Part model, mm, in its own coordinate system. A direction names the side the tool comes from. Round coordinates to 2 decimals unless told otherwise and drop trailing zeros. Loops run counter-clockwise (first coordinate to the right, second up) from the corner with the lowest first, then second, coordinate; pieces in that order, holes last. Notation, with made-up numbers: (-18, -7) - (8, -7) arc R22 ccw to (8, 8) - close; hole circle Ø2 at (-31, 72). An arc over 180 degrees is marked (long way). Put each result on its own line as item: value.
Autodesk Inventor part; units mm, degrees
ref_plane "YZ Plane" through (0, 0, 0) normal (1, 0, 0) x (0, 1, 0)
ref_plane "XZ Plane" through (0, 0, 0) normal (0, 1, 0) x (-1, 0, 0)
ref_plane "XY Plane" through (0, 0, 0) normal (0, 0, 1) x (1, 0, 0)
sketch "Sketch1" plane through (0, 0, 0) normal (0, 0, 1) x (1, 0, 0)
  line L0 (0, 0) -> (50, 0)
  line L1 (50, 0) -> (50, 150)
  line L2 (50, 150) -> (0, 150)
  line L3 (0, 150) -> (0, 0)
  dimension "d0" = 50
  dimension "d1" = 150
extrude "Plate1" add sketch "Sketch1" along normal blind 1
sketch "Sketch2" plane through (50, 149, 1) normal (0, 1, 0) x (-1, 0, 0)
  line L0 (50, 0) -> (0, 0)
  line L1 (0, 0) -> (0, -79)
  line L2 (0, -79) -> (50, -79)
  line L3 (50, -79) -> (50, 0)
edge flange "Flange1" height 79 angle 90 thickness 1 bend radius 1 thickness toward (0, 1, 0) relief tear relief width 1 relief depth 0.5 edges at (25, 150, 0) wall of the first edge with corners at (0, 149, 1) (50, 149, 1) (50, 149, -78) (0, 149, -78)
bend "Bend1"
corner "Corner1"
sketch "Sketch4" plane through (0, 150, -78) normal (0, 1, 0) x (1, 0, 0)
  line L0 (0, 0) -> (50, 0)
  line L1 (0, 0) -> (-40, 0)
  line L2 (-40, 0) -> (-40, -40)
  line L3 (-40, -40) -> (0, -40)
  line L4 (0, -40) -> (0, 0)
  line L5 (50, -77) -> (50, 0)
  line L6 (50, 0) -> (90, 0)
  line L7 (90, 0) -> (90, -40)
  line L8 (90, -40) -> (50, -40)
  line L9 (50, -40) -> (50, 0)
  point P0 (0, -78)
  dimension "d14" = 40
  dimension "d15" = 40
  dimension "d16" = 40
  dimension "d17" = 40
sheet face with bend "Face2" sketch "Sketch4" thickness 1 toward (0, -1, 0) bend radius 1
bend "Bend2"
fillet "Corner Round7" radius 6 2 edges at (50, 149.5, -38) (0, 149.5, -38)
sketch "Sketch3" plane through (0, 150, -78) normal (0, 1, 0) x (1, 0, 0)
  line L0 (0, 0) -> (50, 0)
  circle A0 centre (25, 0) radius 45.5
  arc A1 (-16.7744, -26.5) -> (66.7744, -26.5) centre (25, 0) ccw
  arc A2 (0, -46) -> (-6, -40) centre (-6, -46) ccw
  circle A3 centre (-6, -46) radius 6
  arc A4 (56, -40) -> (50, -46) centre (56, -46) ccw
  circle A5 centre (56, -46) radius 6
  line L1 (-40, -40) -> (-6, -40)
  line L2 (-6, -40) -> (-40, -40)
  line L3 (-40, 0) -> (-40, -40)
  line L4 (-40, -40) -> (-40, 0)
  line L5 (-40, 0) -> (-20.5, 0)
  line L6 (90, 0) -> (-40, 0)
  line L7 (56, -40) -> (90, -40)
  line L8 (56, -40) -> (90, -40)
  line L9 (90, -40) -> (90, 0)
  line L10 (90, -40) -> (90, 0)
  line L11 (90, 0) -> (70.5, 0)
  line L12 (25, 0) -> (25, -45.5)
  line L13 (25, -45.5) -> (25, -23.5) construction
  line L14 (25, -23.5) -> (63.9615, -23.5) construction
  line L15 (63.9615, -23.5) -> (69.9615, -23.5)
  line L16 (63.9615, -23.5) -> (69.9615, -23.5) construction
  line L17 (71.9615, -25.5) -> (71.9615, -30)
  line L18 (70.4615, -31.5) -> (70.4615, -31.5)
  line L19 (25, -23.5) -> (-13.9615, -23.5) construction
  line L20 (-13.9615, -23.5) -> (-19.9615, -23.5)
  line L21 (-13.9615, -23.5) -> (-7.9615, -23.5) construction
  line L22 (-21.9615, -25.5) -> (-21.9615, -30)
  line L23 (-20.4615, -31.5) -> (-20.4615, -31.5)
  arc A6 (-16.7744, -26.5) -> (66.7744, -26.5) centre (25, 0) ccw
  line L24 (-18.9615, -30) -> (-18.9615, -27.5)
  line L25 (-17.9615, -26.5) -> (-16.7744, -26.5)
  line L26 (68.9615, -30) -> (68.9615, -27.5)
  line L27 (67.9615, -26.5) -> (66.7744, -26.5)
  arc A7 (-19.9615, -23.5) -> (-21.9615, -25.5) centre (-19.9615, -25.5) ccw
  arc A8 (-21.9615, -30) -> (-20.4615, -31.5) centre (-20.4615, -30) ccw
  arc A9 (-20.4615, -31.5) -> (-18.9615, -30) centre (-20.4615, -30) ccw
  arc A10 (-17.9615, -26.5) -> (-18.9615, -27.5) centre (-17.9615, -27.5) ccw
  arc A11 (71.9615, -25.5) -> (69.9615, -23.5) centre (69.9615, -25.5) ccw
  arc A12 (70.4615, -31.5) -> (71.9615, -30) centre (70.4615, -30) ccw
  arc A13 (68.9615, -30) -> (70.4615, -31.5) centre (70.4615, -30) ccw
  arc A14 (68.9615, -27.5) -> (67.9615, -26.5) centre (67.9615, -27.5) ccw
  point P0 (0, -78)
  point P1 (52.6469, -41.0244)
  point P2 (-2.6469, -41.0244)
  point P3 (71.9615, -23.5)
  point P4 (71.9615, -31.5)
  point P5 (68.9615, -31.5)
  point P6 (-21.9615, -23.5)
  point P7 (-21.9615, -31.5)
  point P8 (-18.9615, -31.5)
  point P9 (-18.9615, -26.5)
  point P10 (68.9615, -26.5)
  point P11 (-2.6469, -41.0244)
  point P12 (52.6469, -41.0244)
  point P13 (70.4615, -31.5)
  dimension "d13" = 91
  dimension "d84" = 22
  dimension "d85" = 8
  dimension "d86" = 0
  dimension "d87" = 8
  dimension "d88" = 3
  dimension "d89" = 8
  dimension "d90" = 180
  dimension "d91" = 8
  dimension "d92" = 90
  dimension "d93" = 3
  dimension "d95" = 5
  dimension "d96" = 5
  dimension "d97" = 2
  dimension "d98" = 1.5
  dimension "d99" = 1.5
  dimension "d100" = 1
  dimension "d101" = 2
  dimension "d102" = 1.5
  dimension "d103" = 1
extrude "Extrusion1" cut sketch "Sketch3" against normal through all contours L6 A0 L0 | L0 L12 A0 L6 | L0 L6 A0 L12 | A0 L20 A7 L22 A8 A9 L24 A10 L25 A1 A2 L1 L3 L5 | L6 L9 L7 A4 A1 L27 A14 L26 A13 A12 L17 A11 L15 A0
sketch "Sketch5" plane through (0, 150, -1) normal (0, 1, 0) x (1, 0, 0)
  arc A0 (-13.9615, 53.5) -> (63.9615, 53.5) centre (25, 77) ccw
  point P0 (0, -1)
  point P1 (70.5, 77)
  point P2 (-20.5, 77)
sketch "Sketch7" plane through (0, 0, 1) normal (0, 0, 1) x (1, 0, 0)
  line L0 (50, 0) -> (0, 0)
  line L1 (0, 0) -> (0, 148)
  line L2 (50, 148) -> (50, 0)
  point P0 (8, 30)
  point P1 (42, 30)
  dimension "d37" = 30
  dimension "d38" = 8
  dimension "d39" = 8
hole "Hole1" at (8, 30, 1) at (42, 30, 1) direction (0, 0, -1) diameter 4.5 end through all
fillet "Corner Round12" radius 1 1 edges at (-16.7744, 149.5, -51.5)
fillet "Corner Round13" radius 1 1 edges at (66.7744, 149.5, -51.5)
fillet "Corner Round14" radius 3 1 edges at (63.9615, 149.5, -54.5)
fillet "Corner Round15" radius 3 1 edges at (-13.9615, 149.5, -54.5)
sketch "Sketch10" plane through (0, 150, -1) normal (0, 1, 0) x (1, 0, 0)
  arc A0 (70.7921, 70.1608) -> (-20.7921, 70.1608) centre (25, 77) ccw
  line L0 (25, 77) -> (25, 30.7) construction
  line L1 (-17.3207, 50.5) -> (-17.9615, 50.5)
  line L2 (-18.9615, 47) -> (-18.9615, 49.5)
  line L3 (-17.6615, 49.2) -> (-20.7921, 70.1608)
  line L4 (-20.7921, 70.1608) -> (25, 70.1608) construction
  line L5 (68.9615, 49.5) -> (68.9615, 47)
  line L6 (67.3207, 50.5) -> (67.9615, 50.5)
  line L7 (67.6615, 49.2) -> (70.7921, 70.1608)
  line L8 (70.7921, 70.1608) -> (25, 70.1608) construction
  point P0 (0, -1)
  dimension "d109" = 92.6
  dimension "d115" = 1.3
  dimension "d116" = 1.3
  dimension "d117" = 45.7921
  dimension "d118" = 6.8392
  dimension "d119" = 1.3
  dimension "d120" = 1.3
  dimension "d121" = 45.7921
equation "\"d16\" = d14"
equation "\"d17\" = d15"
equation "\"d45\" = Thickness"
equation "\"d2\" = Thickness"
equation "\"d3\" = BendReliefWidth"
equation "\"d4\" = BendReliefDepth"
equation "\"d5\" = MinimumRemnant"
equation "\"d6\" = TransitionRadius"
equation "\"d9\" = BendRadius"
equation "\"d10\" = CornerReliefSize"
equation "\"d11\" = GapSize"
equation "\"d12\" = JacobiRadiusSize"
equation "\"d18\" = BendRadius"
equation "\"d19\" = BendReliefWidth"
equation "\"d21\" = MinimumRemnant"
equation "\"d20\" = BendReliefDepth"
equation "\"d22\" = TransitionRadius"
equation "\"BendRadius\" = Thickness"
equation "\"BendReliefWidth\" = Thickness"
equation "\"BendReliefDepth\" = 0.5 * Thickness"
equation "\"CornerReliefSize\" = 4 * Thickness"
equation "\"MinimumRemnant\" = 2 * Thickness"
equation "\"TransitionRadius\" = BendRadius"
equation "\"JacobiRadiusSize\" = BendRadius"
equation "\"GapSize\" = Thickness"
properties part number "Glass fixer plate" material "Steel, Carbon"
1. Band-saw the part on A-A (y = 30). List the corners of the cut face in (x, z).
A:
outline: (0, 0) - (5.75, 0) - (5.75, 1) - (0, 1) - close; (10.25, 0) - (39.75, 0) - (39.75, 1) - (10.25, 1) - close; (44.25, 0) - (50, 0) - (50, 1) - (44.25, 1) - close
2. Pin check, flat tips, straight feed: P1, Ø0.5, axis at x = 67.5, y = 149.5, coming from the +Z side; P2, Ø15, axis at x = 18.5, y = 55.5, coming from the -Z side; P3, Ø10, axis at x = 54, z = -5, coming from the -Y side; P4, Ø3.5, axis at x = 8, y = 30, coming from the -Z side. Stop position of each tip, or through.
A:
P1: stops at z = -51.5
P2: stops at z = 0
P3: stops at y = 149
P4: passes through
3. Band-saw the part on B-B (z = -40.5). List the corners of the cut face in (x, y), plus the area to 3 significant figures.
A:
outline: (-7.27, 149) - (-0.77, 149) - (-0.77, 150) - (-7.27, 150) - close; (50.77, 149) - (57.27, 149) - (57.27, 150) - (50.77, 150) - close
area: 13.0 mm²
4. Band-saw the part on C-C (x = 8). List the corners of the cut face in (y, z).
A:
outline: (0, 0) - (27.75, 0) - (27.75, 1) - (0, 1) - close; (32.25, 0) - (148, 0) arc R1 cw to (149, -1) - (149, -35.8) - (150, -35.8) - (150, -1) arc R2 ccw to (148, 1) - (32.25, 1) - close
5. Band-saw the part on D-D (x = 27). List the corners of the cut face in (y, z), plus the area to 3 significant figures.
A:
outline: (0, 0) - (148, 0) arc R1 cw to (149, -1) - (149, -32.54) - (150, -32.54) - (150, -1) arc R2 ccw to (148, 1) - (0, 1) - close
area: 182 mm²
6. Tool access for faces 5 (the cylindrical face through (60.175, 149.507, -43.214)), 6 (the cylindrical face through (40.103, 28.79, 0.493)), 7 (the flat face through (26, 149, -21)): list every direction of +Z, -Z, +X, -X, +Y, -Y with a clear straight run to the whole face (end or side of a thin tool).
A:
face 5: +Z, +Y, -Y
face 6: +Z, -Z
face 7: -Z, +X, -X, -Y
7. Two-plate mould, pull along X, no slides. Class faces 1 (the cylindrical face through (24.368, 149.507, -32.504)), 2 (the cylindrical face through (-10.37, 149.51, -43.41)), 3 (the flat face through (25, 75, 0)), 4 (the flat face through (0, 75.4, 0.3)): pulls with the +X half, pulls with the -X half, needs draft (parallel to the pull), parting line crosses it, or undercut.
A:
face 1: undercut
face 2: undercut
face 3: needs draft
face 4: pulls with the -X half
8. Probe line 1 along X through (y, z) = (30, 0.6); line 2 along Z through (x, y) = (34, 106.5); line 3 along Y through (x, z) = (58, -42.5). List the from-to ranges inside material, lowest first. Write a range as [from, to].
A:
line 1: x = [0, 5.75], [10.25, 39.75], [44.25, 50]
line 2: z = [0, 1]
line 3: y = [149, 150]
